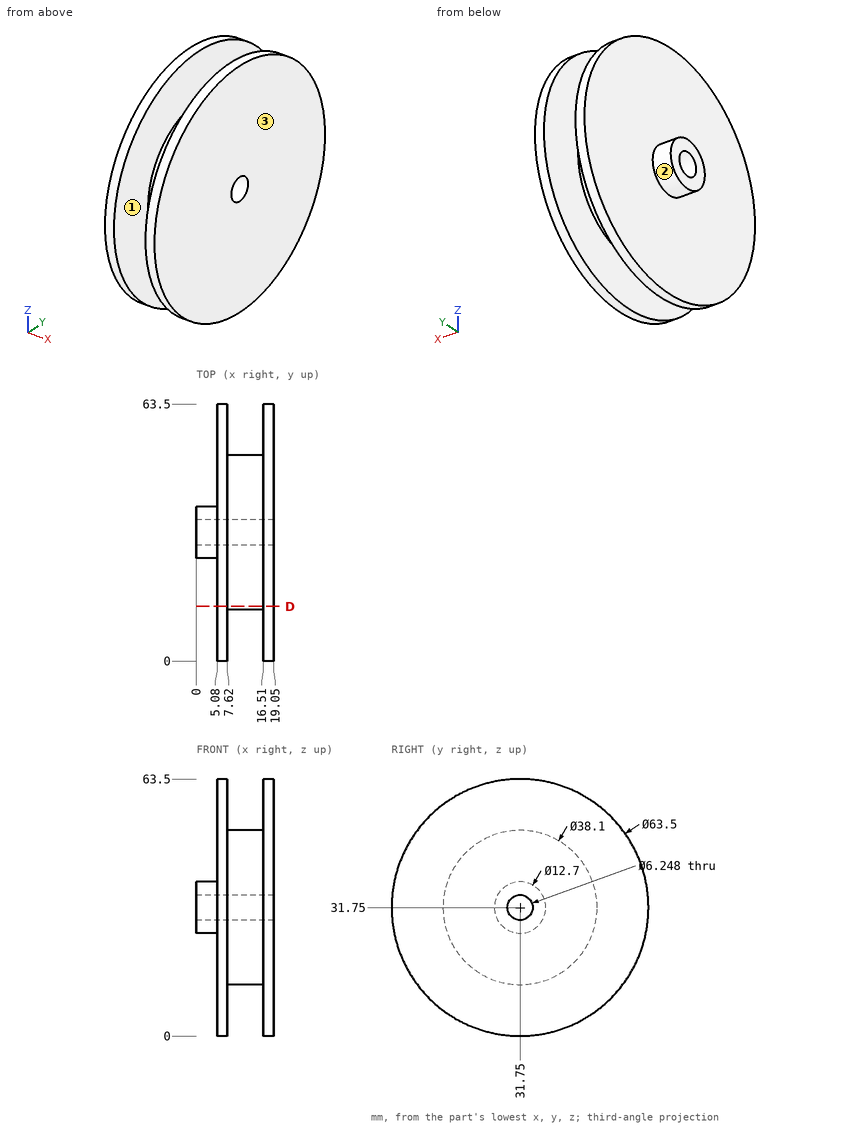
Here's the drawing with two shaded views (mm, measured from the low corner). I have some questions. Coordinates: 2 decimals unless noted, no trailing zeros. Write each loop counter-clockwise with the first axis right and the second up, starting at its lowest first coordinate (ties: lowest second). Pieces come first, ordered by that corner, then holes.
Item 1: Will these pins go through, and if not, where does the flat tip stop? pin 1 (6 mm diameter, centred on x = 12, y = 38, fed in from +Z); pin 2 (5 mm diameter, centred on x = 6.5, z = 17.5, fed in from +Y) (1 decimal); pin 3 (8 mm diameter, centred on x = 5, z = 57, fed in from -Y).
Item 2: I want a section at D-D on y = 13.5. Write out the boundary of the cut face in (x, z).
Item 3: If we mould it in two halves opening along X, with no side actions, what happens to the marked faces 1, 2 and 3? For each: +X half, -X half, draft (parallel to the pull), parting line (faces both ways), or undercut.
Item 4: If I drill on line 1 (X direction, y = 45, z = 12); line 2 (Z direction, x = 12.25, y = 31.5) (1 decimal); line 3 (X direction, y = 41, z = 28.5), over which ranges is the centre line in solid material (lowest first)?
Findings below:
1. pin 1: stops at z = 50.52
1. pin 2: stops at y = 61.2
1. pin 3: stops at y = 8.16
2. outline: (5.08, 5.77) - (7.62, 5.77) - (7.62, 26.29) - (16.51, 26.29) - (16.51, 5.77) - (19.05, 5.77) - (19.05, 57.73) - (16.51, 57.73) - (16.51, 37.21) - (7.62, 37.21) - (7.62, 57.73) - (5.08, 57.73) - close
3. face 1: undercut
3. face 2: draft
3. face 3: +X half
4. line 1: x = 5.08 to 7.62, 16.51 to 19.05
4. line 2: z = 12.7 to 28.6, 34.9 to 50.8
4. line 3: x = 5.08 to 19.05
